Build history of the part. All positions in model axes, mm. Give positions to 0.01 mm unless a question says otherwise; leave off trailing zeros. Order: outer loops, then holes, each group sorted by start corner. A loop starts at its lowest first (then second) coordinate and runs counter-clockwise, first axis right, second up. Notation, with made-up numbers: M 24.25,41.25 L 73.25,41.25 A10 ccw 73.25,45.25 Z; hole C 8.25,-20 d5. An arc over 180 degrees is marked long. One line per item, written item: value. Start each with the question number.
from build123d import *

# Parameters (mm, degrees)
SKETCH1_W           = 88.9
SKETCH1_H           = 44.45
BOSS_EXTRUDE1_DEPTH = 1219.2
CUT_EXTRUDE1_DEPTH  = 1221.819497305
SKETCH3_R           = 6.35
CUT_EXTRUDE2_DEPTH  = 22.225
LPATTERN1_COUNT     = 10
LPATTERN1_PITCH     = 101.6


with BuildPart() as part:
    # Sketch1 → Boss-Extrude1 (new body)
    with BuildSketch(Plane.XY):
        Rectangle(SKETCH1_W, SKETCH1_H)
    extrude(amount=BOSS_EXTRUDE1_DEPTH)

    # Sketch2 → Cut-Extrude1 (cut, through all)
    with BuildSketch(Plane(origin=(0, 22.225, 0), x_dir=(1, 0, 0), z_dir=(0, 1, 0))):
        Polygon((-44.45, -1219.2), (0, -1219.2), (-44.45, -1174.75), align=None)
        Polygon((44.45, -1174.75), (0, -1219.2), (44.45, -1219.2), align=None)
    extrude(amount=-CUT_EXTRUDE1_DEPTH, mode=Mode.SUBTRACT)

    # Sketch3 → Cut-Extrude2 (cut)
    with BuildSketch(Plane(origin=(0, 22.225, 0), x_dir=(1, 0, 0), z_dir=(0, 1, 0))):
        with Locations(Location((0, -1117.6, 0), (0, 0, 270))):
            Circle(SKETCH3_R)
    cut_extrude2 = extrude(amount=-CUT_EXTRUDE2_DEPTH, mode=Mode.SUBTRACT)

    # LPattern1: Cut-Extrude2 ×10
    with Locations(*[(0, 0, -i * LPATTERN1_PITCH) for i in range(1, LPATTERN1_COUNT)]):
        add(cut_extrude2, mode=Mode.SUBTRACT)


solid = part.part
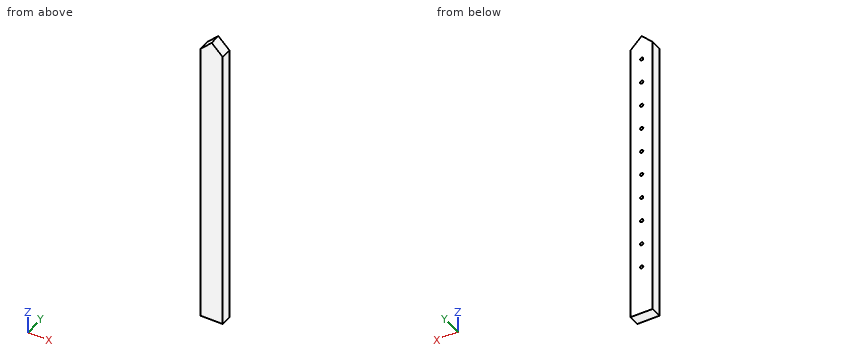
1) Drop a flat-ended pin along its axis: P1, Ø6.5, axis at x = -0.5, z = 407.5, coming from the +Y side. Give the stop position or say it passes through.
2) Slice it at A-A (y = 11). State how many separate pieces and enclosed holes the cut face has, plus the area to 3 significant figures.
3) Slice it at B-B (x = -21.5). List the corners of the cut face in (y, z) (3 decimals).
4) Drill centre lines: line 1 (X direction, y = 9, z = 812.8); line 2 (Y direction, x = 3, z = 712) (3 decimals); line 3 (Z direction, x = -16, y = 6.5). Where is each one in solid material? Low to high.
Results list:
1. P1: stops at y = 0
2. separate pieces: 1
2. enclosed holes: 10
2. area: 105,000 mm²
3. outline: M -22.225,0 L 22.225,0 L 22.225,1197.7 L -22.225,1197.7 Z
4. line 1: x = -44.45 to -6.35, 6.35 to 44.45
4. line 2: y = -22.225 to 0
4. line 3: z = 0 to 1203.2
